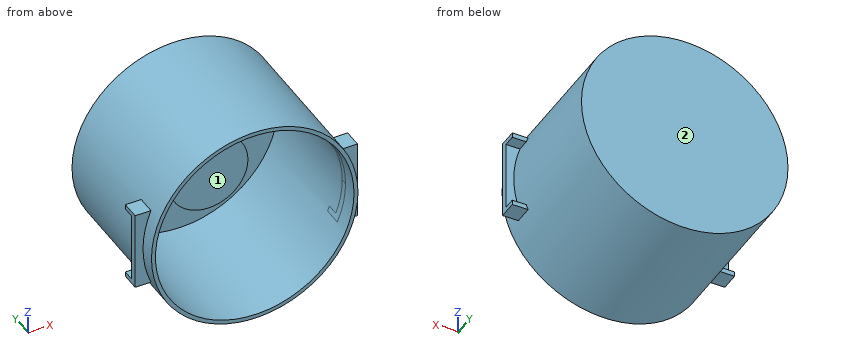
from build123d import *

# Parameters (mm, degrees)
F0_R     = 130
F1_DEPTH = 8
F2_R     = 130
F2_R_2   = 125
F3_DEPTH = 180
F4_R     = 50
F5_DEPTH = 70
F6_W     = 15
F6_H     = 6
F7_DEPTH = 140
F8_DEPTH = 25


with BuildPart() as f1:
    # F0 (on Front) → F1 (new body)
    with BuildSketch(Plane.XZ):
        Circle(F0_R)
    extrude(amount=F1_DEPTH)

    # F2 (on face) → F3 (join)
    with BuildSketch(Plane.XZ.offset(8)):
        Circle(F2_R)
        Circle(F2_R_2, mode=Mode.SUBTRACT)
    extrude(amount=F3_DEPTH)

    # F4 (on face) → F5 (join)
    with BuildSketch(Plane.XZ.offset(8)):
        Circle(F4_R)
    extrude(amount=F5_DEPTH)

    # F6 (on Right) → F7 (join, symmetric)
    with BuildSketch(Plane.YZ):
        Polygon((-160, 50), (-168, 50), (-168, -50), (-160, -50), (-160, -44), (-160, 44), align=None)
        with Locations((-152.5, 47)):
            Rectangle(F6_W, F6_H)
        with Locations((-152.5, -47)):
            Rectangle(F6_W, F6_H)
    extrude(amount=F7_DEPTH, both=True)

    # F7_face (on face) → F8 (cut)
    with BuildSketch(Plane.XZ.offset(168)):
        with BuildLine():
            Line((114.564392, 50), (-114.564392, 50))
            ThreePointArc((-114.564392, 50), (-125, 0), (-114.564392, -50))
            Line((-114.564392, -50), (114.564392, -50))
            ThreePointArc((114.564392, -50), (122.363289, -25.538705), (125, 0))
            ThreePointArc((125, 0), (122.363289, 25.538705), (114.564392, 50))
        make_face()
    extrude(amount=-F8_DEPTH, mode=Mode.SUBTRACT)


solid = f1.part
The model under review builds one solid part; all positions refer to its coordinate system, in mm. Face numbers are marked on the shaded views. Coordinates: 2 decimals unless noted, no trailing zeros. Loops run counter-clockwise (first coordinate to the right, second up) from the corner with the lowest first, then second, coordinate; pieces in that order, holes last. Notation, with made-up numbers: M -33.75,70.5 L -0.75,70.5 A21 ccw -0.75,90.5 Z; hole C -5.5,42.25 d6. An arc over 180 degrees is marked long. Put each result on its own line as item: value. Start each with the question number.
Q1. Add section C-C (z = -89.5). Write out the cut boundary in (x, y), and give its area (3 significant figures).
Q2. Add section D-D (y = -92). Write out the cut boundary in (x, z).
Q3. Wall thickness on line 1 (Z direction, x = 0, y = -44.5); line 2 (Z direction, x = 0, y = -115); line 3 (Y direction, x = -77, z = 34.5): over which ranges is each line inside the solid? List them lowest first.
Q4. Add section A-A (y = -18). Write out the cut boundary in (x, z), and give its area (3 significant figures).
Q5. The part is to be moulded in two halves that separate along Z. For the marked faces 1 and 2, say which applies: +Z half, -Z half, draft (parallel to the pull), parting line (faces both ways), or undercut.
Q6. Clearance check with flat-ended pins moving along their axes: pin 1 (1 mm diameter, centred on x = -45, y = -52, fed in from +Z); pin 2 (5 mm diameter, centred on y = -121.5, z = 50, fed in from -X); pin 3 (16.5 mm diameter, centred on x = -127, y = -152, fed in from +Z); pin 4 (5.5 mm diameter, centred on x = 131, z = 20.5, fed in from +Y). State where each tip first meets the part, or that it passes through.
Q7. Add section B-B (x = 0). Write out the cut boundary in (y, z).
Answers:
1. outline: M -94.29,-188 L -87.26,-188 L -87.26,-8 L 87.26,-8 L 87.26,-188 L 94.29,-188 L 94.29,0 L -94.29,0 Z
1. area: 4,040 mm^2
2. outline: C 0,0 d260; hole C 0,0 d250
3. line 1: z = -130 to -125, -50 to 50, 125 to 130
3. line 2: z = -130 to -125, 125 to 130
3. line 3: y = -8 to 0
4. outline: C 0,0 d260; C 0,0 d100; hole C 0,0 d250
4. area: 11,900 mm^2
5. face 1: undercut
5. face 2: draft
6. pin 1: stops at z = 122.15
6. pin 2: stops at x = -121.01
6. pin 3: stops at z = 52.9
6. pin 4: stops at y = 0
7. outline: M -188,-130 L 0,-130 L 0,130 L -188,130 L -188,125 L -8,125 L -8,50 L -78,50 L -78,-50 L -8,-50 L -8,-125 L -188,-125 Z
